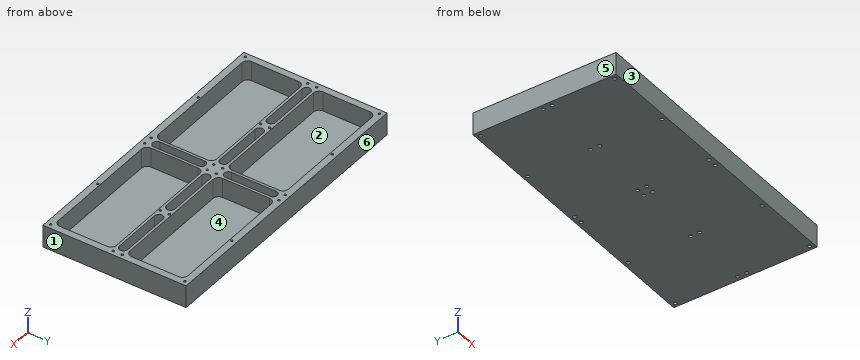
from build123d import *

# Parameters (mm, degrees)
SKIZZE1_W                                            = 512
SKIZZE1_H                                            = 256
AUFSATZ_LINEAR_AUSTRAGEN1_DEPTH                      = 40
SKIZZE2_W                                            = 488
SKIZZE2_H                                            = 232
SCHNITT_LINEAR_AUSTRAGEN1_DEPTH                      = 35
AUFSATZ_LINEAR_AUSTRAGEN2_DEPTH                      = 35
STIRNSENKUNG_F_R_M3_ZYLINDERSCHRAUBE_MIT_D           = 4
STIRNSENKUNG_F_R_M3_ZYLINDERSCHRAUBE_MIT_CBORE_D     = 6.5
STIRNSENKUNG_F_R_M3_ZYLINDERSCHRAUBE_MIT_CBORE_DEPTH = 3.4
VERRUNDUNG1_R                                        = 10
SCHNITT_LINEAR_AUSTRAGEN2_DEPTH                      = 35
SPIEGELN7_COPY_1_DEPTH                               = 35
SCHNITT_LINEAR_AUSTRAGEN3_DEPTH                      = 35


with BuildPart() as part:
    # Skizze1 → Aufsatz-Linear austragen1 (new body)
    with BuildSketch(Plane.XY):
        with Locations((256, 128)):
            Rectangle(SKIZZE1_W, SKIZZE1_H)
    extrude(amount=AUFSATZ_LINEAR_AUSTRAGEN1_DEPTH)

    # Skizze2 → Schnitt-Linear austragen1 (cut)
    with BuildSketch(Plane.XY.offset(40)):
        with Locations((256, 128)):
            Rectangle(SKIZZE2_W, SKIZZE2_H)
    extrude(amount=-SCHNITT_LINEAR_AUSTRAGEN1_DEPTH, mode=Mode.SUBTRACT)

    # Skizze5 → Aufsatz-Linear austragen2 (add)
    with BuildSketch(Plane.XY.offset(5)):
        Polygon((12, 140), (244, 140), (244, 244), (268, 244), (268, 140), (500, 140), (500, 116), (268, 116), (268, 12), (244, 12), (244, 116), (12, 116), align=None)
    extrude(amount=AUFSATZ_LINEAR_AUSTRAGEN2_DEPTH)

    # Stirnsenkung für M3 Zylinderschraube mit Innensechskant1 (through all)
    with Locations(Plane(origin=(0, 0, 0), x_dir=(1, 0, 0), z_dir=(0, 0, -1))):
        with Locations((8, -248), (128, -248), (248, -248), (264, -248), (384, -248), (384, -8), (264, -8), (128, -8), (504, -248), (504, -8), (8, -8), (384, -136), (264, -136), (128, -136), (128, -120), (264, -120), (384, -120), (248, -136), (248, -120), (248, -8), (504, -136), (504, -120), (8, -136), (8, -120)):
            CounterBoreHole(STIRNSENKUNG_F_R_M3_ZYLINDERSCHRAUBE_MIT_D / 2, STIRNSENKUNG_F_R_M3_ZYLINDERSCHRAUBE_MIT_CBORE_D / 2, STIRNSENKUNG_F_R_M3_ZYLINDERSCHRAUBE_MIT_CBORE_DEPTH)

    # Verrundung1
    verrundung1_edges = [part.edges().sort_by_distance(p)[0] for p in [
        (12, 244, 22.5),
        (500, 244, 22.5),
        (500, 12, 22.5),
        (12, 12, 22.5),
        (244, 140, 22.5),
        (244, 244, 22.5),
        (268, 244, 22.5),
        (268, 140, 22.5),
        (500, 140, 22.5),
        (500, 116, 22.5),
        (268, 116, 22.5),
        (268, 12, 22.5),
        (244, 12, 22.5),
        (244, 116, 22.5),
        (12, 116, 22.5),
        (12, 140, 22.5),
    ]]
    fillet(verrundung1_edges, radius=VERRUNDUNG1_R)

    # Skizze6 → Schnitt-Linear austragen2 (cut)
    with BuildSketch(Plane.XY.offset(40)):
        with BuildLine():
            Line((489, 120.5), (399, 120.5))
            ThreePointArc((399, 120.5), (391.5, 128), (399, 135.5))
            Line((399, 135.5), (489, 135.5))
            ThreePointArc((489, 135.5), (496.5, 128), (489, 120.5))
        make_face()
    schnitt_linear_austragen2 = extrude(amount=-SCHNITT_LINEAR_AUSTRAGEN2_DEPTH, mode=Mode.SUBTRACT)

    # Skizzen-Muster1: Schnitt-Linear austragen2 at 1 more place
    with Locations((-120, 0, 0)):
        add(schnitt_linear_austragen2, mode=Mode.SUBTRACT)

    # Spiegeln7: Schnitt-Linear austragen2 across plane
    add(schnitt_linear_austragen2.mirror(Plane.ZY.offset(-256)), mode=Mode.SUBTRACT)

    # Spiegeln7 copy 1 sketch → Spiegeln7 copy 1 (cut)
    with BuildSketch(Plane(origin=(632, 0, 40), x_dir=(-1, 0, 0), z_dir=(0, 0, 1))):
        with BuildLine():
            Line((489, -120.5), (399, -120.5))
            ThreePointArc((399, -120.5), (391.5, -128), (399, -135.5))
            Line((399, -135.5), (489, -135.5))
            ThreePointArc((489, -135.5), (496.5, -128), (489, -120.5))
        make_face()
    extrude(amount=-SPIEGELN7_COPY_1_DEPTH, mode=Mode.SUBTRACT)

    # Skizze9 → Schnitt-Linear austragen3 (cut)
    with BuildSketch(Plane.XY.offset(40)):
        with BuildLine():
            Line((263.5, 232), (263.5, 152))
            ThreePointArc((263.5, 152), (256, 144.5), (248.5, 152))
            Line((248.5, 152), (248.5, 232))
            ThreePointArc((248.5, 232), (256, 239.5), (263.5, 232))
        make_face()
    schnitt_linear_austragen3 = extrude(amount=-SCHNITT_LINEAR_AUSTRAGEN3_DEPTH, mode=Mode.SUBTRACT)

    # Spiegeln8: Schnitt-Linear austragen3 across plane
    add(schnitt_linear_austragen3.mirror(Plane.ZX.offset(128)), mode=Mode.SUBTRACT)


solid = part.part
Verification items for the finished model (mm, model axes). Face numbers are marked on the shaded views. A direction names the side the tool comes from. Give positions to 0.01 mm unless a question says otherwise; leave off trailing zeros. Write each loop counter-clockwise with the first axis right and the second up, starting at its lowest first coordinate (ties: lowest second). Pieces come first, ordered by that corner, then holes.
(1) Cross-section at C-C (z = 17). State how many separate pieces and enclosed holes the cut face has, plus the area to 3 significant figures.
(2) Cross-section at B-B (y = 189.5). Enter the section's corners in (x, z).
(3) Material ranges on line 1 (X direction, y = 182, z = 26.5); line 2 (Y direction, x = 8, z = 31); line 3 (Y direction, x = 384, z = 1.1), recorded low to high.
(4) Cross-section at A-A (x = 256). Enter the section's corners in (y, z), plus the area to 3 significant figures.
(5) Gauge pin test, flat end, axial feed: pin 1 (2 mm diameter, centred on x = 128, y = 9.5, fed in from -Z). Record the tip position at first contact, or that the pin passes through.
(6) Mould release check, pull along Y, two halves, no side actions. Record for the marked faces 3, 4, 5 and 6: +Y half, -Y half, draft (parallel to the pull), parting line (faces both ways), or undercut.
(7) Access from +Z, -Z, +X, -X, +Y, -Y to the whole of each face (thin tool, end or side, straight path). Record for the marked faces 1 and 2.
Worked out:
1. separate pieces: 1
1. enclosed holes: 34
1. area: 25,700 mm2
2. outline: (0, 0) - (512, 0) - (512, 40) - (500, 40) - (500, 5) - (268, 5) - (268, 40) - (263.5, 40) - (263.5, 5) - (248.5, 5) - (248.5, 40) - (244, 40) - (244, 5) - (12, 5) - (12, 40) - (0, 40) - close
3. line 1: x = 0 to 12, 244 to 248.5, 263.5 to 268, 500 to 512
3. line 2: y = 0 to 6, 10 to 118, 122 to 134, 138 to 246, 250 to 256
3. line 3: y = 0 to 4.75, 11.25 to 116.75, 123.25 to 132.75, 139.25 to 244.75, 251.25 to 256
4. outline: (0, 0) - (256, 0) - (256, 40) - (239.5, 40) - (239.5, 5) - (144.5, 5) - (144.5, 40) - (111.5, 40) - (111.5, 5) - (16.5, 5) - (16.5, 40) - (0, 40) - close
4. area: 3,590 mm2
5. pin 1: stops at z = 3.4
6. face 3: -Y half
6. face 4: undercut
6. face 5: draft
6. face 6: +Y half
7. face 1: +Z, -Z, +X, +Y, -Y
7. face 2: +Z
